Here's how the part is built. I have some questions about the finished solid (model axes, mm). Face numbers are marked on the shaded views. Give positions to 0.01 mm unless a question says otherwise; leave off trailing zeros. Write each loop counter-clockwise with the first axis right and the second up, starting at its lowest first coordinate (ties: lowest second). Pieces come first, ordered by that corner, then holes. Notation, with made-up numbers: M -36,-35.5 L -10,-35.5 A25 cw -10,-21.5 Z; hole C -35,13.25 d6. An arc over 180 degrees is marked long. Use one line per item in the form item = value. Start each with the question number.
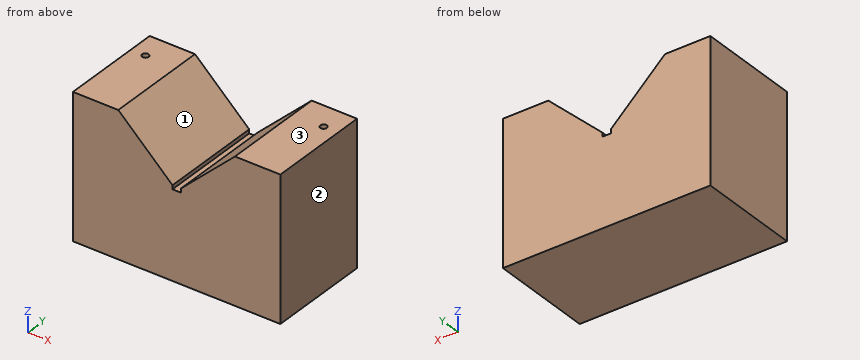
from build123d import *

# Parameters (mm, degrees)
F0_W     = 203.2
F0_H     = 139.7
F1_DEPTH = 50.8
F3_DEPTH = 101.601
F5_DEPTH = 101.601
F6_R     = 3.2385
F7_DEPTH = 23.8125


with BuildPart() as f1:
    # F0 (on Front) → F1 (new body, symmetric)
    with BuildSketch(Plane.XZ):
        with Locations((0, 69.85)):
            Rectangle(F0_W, F0_H)
    extrude(amount=F1_DEPTH, both=True)

    # F2 (on face) → F3 (cut, through all)
    with BuildSketch(Plane.XZ.offset(50.8)):
        Polygon((57.15, 139.7), (0, 139.7), (0, 85.725), align=None)
        Polygon((0, 85.725), (0, 139.7), (-57.15, 139.7), align=None)
    extrude(amount=-F3_DEPTH, mode=Mode.SUBTRACT)

    # F4 (on face) → F5 (cut, through all)
    with BuildSketch(Plane.XZ.offset(50.8)):
        Polygon((-4.064, 90.043), (-4.064, 85.725), (4.064, 85.725), (4.064, 90.043), (0, 90.043), align=None)
    extrude(amount=-F5_DEPTH, mode=Mode.SUBTRACT)

    # F6 (on face) → F7 (cut)
    with BuildSketch(Plane.XY.offset(139.7)):
        with Locations((-87.3125, 25.8445)):
            Circle(F6_R)
        with Locations((87.3125, 25.8445)):
            Circle(F6_R)
    extrude(amount=-F7_DEPTH, mode=Mode.SUBTRACT)


solid = f1.part
1) Will these pins go through, and if not, where does the flat tip stop? P1, Ø9, axis at x = 1.5, y = -17.5, coming from the +Z side; P2, Ø10, axis at x = -27.5, y = -30.5, coming from the +Z side; P3, Ø3, axis at x = 88, y = 27, coming from the +Z side.
2) Suppose I cut it at D-D, the plane x = -33.5. List the corners of the cut face in (y, z) for me.
3) Suppose I cut it at A-A, the plane y = -25. List the corners of the cut face in (x, z) for me (3 decimals).
4) Suppose I cut it at B-B, the plane z = 104.5. List the corners of the cut face in (x, y) for me.
5) Suppose I cut it at C-C, the plane x = 54. List the corners of the cut face in (y, z) for me (3 decimals), and give its area (3 significant figures).
6) Thinking about a two-plate mould opening in X: for the marked faces 1, 2 and 3, which applies, released by +X, released by -X, zero draft, split by the parting line, or undercut?
7) Please list where these lines run through material, in increasing order: line 1 (X direction, y = 28, z = 122); line 2 (X direction, y = -1.5, z = 127.5); line 3 (Z direction, x = -1.5, y = 22) (3 decimals).
Checks:
q1.P1 = 91.39
q1.P2 = 116.42
q1.P3 = 115.89
q2.outline = M -50.8,0 L 50.8,0 L 50.8,117.36 L -50.8,117.36 Z
q3.outline = M -101.6,0 L 101.6,0 L 101.6,139.7 L 57.15,139.7 L 4.064,89.563 L 4.064,85.725 L -4.064,85.725 L -4.064,89.563 L -57.15,139.7 L -101.6,139.7 Z
q4.outline = M -101.6,-50.8 L -19.88,-50.8 L -19.88,50.8 L -101.6,50.8 Z; M 19.88,-50.8 L 101.6,-50.8 L 101.6,50.8 L 19.88,50.8 Z
q5.outline = M -50.8,0 L 50.8,0 L 50.8,136.725 L -50.8,136.725 Z
q5.area = 13,900 mm^2
q6.face_1 = undercut
q6.face_2 = released by +X
q6.face_3 = zero draft
q7.line_1 = -101.6 to -89.73, -84.9 to -38.41, 38.41 to 84.9, 89.73 to 101.6
q7.line_2 = -101.6 to -44.23, 44.23 to 101.6
q7.line_3 = 0 to 85.725
